```python
from build123d import *

# Parameters (mm, degrees)
F0_R     = 31.75
F1_DEPTH = 3.556
F3_D     = 58.42
F3_DEPTH = 5.08
F3_TIP   = 17.5511386818
F4_R     = 1.26999


# Not quite as in the source:
# - a fillet or chamfer is up to 0.001 mm smaller than in the source, because OpenCascade refuses the exact size


with BuildPart() as f1:
    # F0 (on Top) → F1 (new body)
    with BuildSketch(Plane.XY):
        Circle(F0_R)
    extrude(amount=F1_DEPTH)

    # F3
    with Locations(Plane.XY.offset(3.556)):
        with Locations((0, 0)):
            Hole(F3_D / 2, depth=F3_DEPTH)
            with Locations((0, 0, -(F3_DEPTH + F3_TIP / 2))):  # 118° drill point
                Cone(0, F3_D / 2, F3_TIP, mode=Mode.SUBTRACT)

    # F4 (radius 1.27 in the source; OpenCascade refuses exactly that, so slightly less here)
    f4_edges = [f1.edges().sort_by_distance(p)[0] for p in [
        (-31.75, 0, 0),
        (-31.75, 0, 3.556),
        (-29.21, 0, 0),
        (-29.21, 0, 3.556),
    ]]
    fillet(f4_edges, radius=F4_R)


solid = f1.part
```
Geometry: final body of the model. Coordinates: model frame, mm. Coordinates: 2 decimals unless noted, no trailing zeros. Put each result on its own line as item: value.
(1) Draft query along X for faces 1 (the face through (21.53, 19.74, 1.77)), 2 (the face through (-6.883, -30.995, 1.771)). Return one class per face: pulls with the +X half, pulls with the -X half, needs draft (parallel to the pull), parting line crosses it, or undercut.
Answer sheet:
face 1: undercut
face 2: parting line crosses it
(2) First-contact query: pin 1 (2 mm diameter, centred on y = -15.5, z = 0.5, fed in from -X); pin 2 (10 mm diameter, centred on x = 24, y = 6.5, fed in from -Z). Flat tips, straight axial feed; report the tip coordinate or a pass-through.
Answer sheet:
pin 1: stops at x = -28.14
pin 2: stops at z = 0.16
(3) Material intervals for probe 1 along Y at (x, z) = (0, 1.75); probe 2 along Y at (x, z) = (26, 0.6); probe 3 along X at (y, z) = (5, 0.3), sorted ascending.
Answer sheet:
probe 1: y = -31.75 to -29.21, 29.21 to 31.75
probe 2: y = -17.89 to -13.73, 13.73 to 17.89
probe 3: x = -30.9 to -29.24, 29.24 to 30.9
